Geometry: final body of the model. Coordinates: model frame, mm. Give positions to 0.01 mm unless a question says otherwise; leave off trailing zeros. Write each loop counter-clockwise with the first axis right and the second up, starting at its lowest first coordinate (ties: lowest second). Pieces come first, ordered by that corner, then holes. Notation, with made-up numbers: (68, 39) -> (105, 39) arc R21 ccw to (105, 59) -> close; hole circle Ø10 at (76.5, 73). An arc over 180 degrees is marked (long way). Use CSV: the item, a comma, the result in double quotes. Start each with the question number.
1) Contact query for flat-ended pins moving along their axis: P1, Ø3, axis at y = 11, z = 9.5, coming from the +X side; P2, Ø15.5, axis at x = 0, y = 0, coming from the +Z side; P3, Ø1.5, axis at x = 7.5, z = 6, coming from the -Y side; P4, Ø6, axis at y = -7.5, z = 6, coming from the -X side. Output: stop coordinate, or through.
2) Draft query along Z for faces 1 (the face through (13.3, 0.3, 0)), 2 (the face through (-3.414, -15.374, 7.842)), 3 (the face through (2.808, -12.646, 7.776)), 4 (the face through (13.3, 0.3, 15.773)). Return one class per face: pulls with the +Z half, pulls with the -Z half, needs draft (parallel to the pull), parting line crosses it, or undercut.
3) Section B-B (z = 10). Output: boundary loops of the cut face in (x, y).
4) Material intervals for line 1 (Y direction, x = 0, z = 6.75); line 2 (Z direction, x = 11.5, y = -11.5); line 3 (Y direction, x = 0, z = 3), sorted ascending. Write a range as [from, to].
5) Section A-A (x = 0). Output: boundary loops of the cut face in (y, z).
6) Section C-C (z = 3.5). Output: boundary loops of the cut face in (x, y).
```python
from build123d import *

# Parameters (mm, degrees)
F0_R      = 20.3835
F2_R      = 15.748
F4_DEPTH  = 6.4262
F6_R      = 20.3835
F4_FACE_R = 15.748
F9_D      = 25.908


with BuildPart() as f3:
    # F0 (on Top) → F3 section 0
    with BuildSketch(Plane.XY):
        Circle(F0_R)
    # F2 (on offset) → F3 section 1
    with BuildSketch(Plane.XY.offset(4.6736)):
        Circle(F2_R)
    loft()

    # F4 (add): a face of the model
    f4_faces = [f3.faces().sort_by_distance(p)[0] for p in [
        (0, 0, 4.6736),
    ]]
    extrude(f4_faces, amount=F4_DEPTH)

    # F6 (on offset) → F7 section 0
    with BuildSketch(Plane.XY.offset(15.7734)):
        Circle(F6_R)
    # F4_face (on face) → F7 section 1
    with BuildSketch(Plane.XY.offset(11.0998)):
        Circle(F4_FACE_R)
    loft()

    # F9 (through all)
    with Locations(Plane.XY.offset(15.7734)):
        with Locations((0, 0)):
            Hole(F9_D / 2)


solid = f3.part
```
Answers follow:
1,P1,"stops at x = 12.56"
1,P2,"passes through"
1,P3,"stops at y = -14.23"
1,P4,"stops at x = -15.97"
2,face 1,"pulls with the -Z half"
2,face 2,"undercut"
2,face 3,"needs draft"
2,face 4,"pulls with the +Z half"
3,outline,"circle Ø31.5 at (0, 0); hole circle Ø25.91 at (0, 0)"
4,line 1,"y = [-15.75, -12.95], [12.95, 15.75]"
4,line 2,"z = [0, 4.15], [11.62, 15.77]"
4,line 3,"y = [-17.41, -12.95], [12.95, 17.41]"
5,outline,"(-20.38, 0) -> (-12.95, 0) -> (-12.95, 15.77) -> (-20.38, 15.77) -> (-15.75, 11.1) -> (-15.75, 4.67) -> close; (12.95, 0) -> (20.38, 0) -> (15.75, 4.67) -> (15.75, 11.1) -> (20.38, 15.77) -> (12.95, 15.77) -> close"
6,outline,"circle Ø33.82 at (0, 0); hole circle Ø25.91 at (0, 0)"
